For this review, take the finished solid that the model builds, in its own axes (mm). Face numbers are marked on the shaded views. A direction names the side the tool comes from. Round coordinates to 2 decimals unless told otherwise and drop trailing zeros. Order: outer loops, then holes, each group sorted by start corner. A loop starts at its lowest first (then second) coordinate and runs counter-clockwise, first axis right, second up. Notation, with made-up numbers: (29, 42.5) -> (80, 42.5) arc R16 cw to (80, 64.5) -> close; hole circle Ø11 at (40, 48.25). An arc over 180 degrees is marked (long way). Answer in a Markdown table with one row per item.
```python
from build123d import *

# Parameters (mm, degrees)
SKIZZE1_W                       = 140
SKIZZE1_H                       = 210
AUFSATZ_LINEAR_AUSTRAGEN1_DEPTH = 2
SKIZZE2_W                       = 20
SKIZZE2_H                       = 210
AUFSATZ_LINEAR_AUSTRAGEN2_DEPTH = 15
SKIZZE3_W                       = 94.4
SKIZZE3_H                       = 56
SCHNITT_LINEAR_AUSTRAGEN1_DEPTH = 10
VERRUNDUNG1_R                   = 1


with BuildPart() as part:
    # Skizze1 → Aufsatz-Linear austragen1 (new body)
    with BuildSketch(Plane(origin=(0, 0, 0), x_dir=(1, 0, 0), z_dir=(0, 1, 0))):
        Rectangle(SKIZZE1_W, SKIZZE1_H)
    extrude(amount=AUFSATZ_LINEAR_AUSTRAGEN1_DEPTH)

    # Skizze2 → Aufsatz-Linear austragen2 (add)
    with BuildSketch(Plane(origin=(0, 2, 0), x_dir=(1, 0, 0), z_dir=(0, 1, 0))):
        with Locations((-46.2, 0)):
            Rectangle(SKIZZE2_W, SKIZZE2_H)
        with Locations((46.2, 0)):
            Rectangle(SKIZZE2_W, SKIZZE2_H)
    extrude(amount=AUFSATZ_LINEAR_AUSTRAGEN2_DEPTH)

    # Skizze3 → Schnitt-Linear austragen1 (cut)
    with BuildSketch(Plane(origin=(0, 17, 0), x_dir=(1, 0, 0), z_dir=(0, 1, 0))):
        Rectangle(SKIZZE3_W, SKIZZE3_H)
        with Locations((0, -68)):
            Rectangle(SKIZZE3_W, SKIZZE3_H)
        with Locations((0, 68)):
            Rectangle(SKIZZE3_W, SKIZZE3_H)
    extrude(amount=-SCHNITT_LINEAR_AUSTRAGEN1_DEPTH, mode=Mode.SUBTRACT)

    # Verrundung1
    verrundung1_edges = [part.edges().sort_by_distance(p)[0] for p in [
        (41.7, 17, 28),
        (41.7, 17, -40),
        (41.7, 17, 96),
        (36.2, 7, 0),
        (36.2, 7, -68),
        (36.2, 7, 68),
        (-36.2, 7, 68),
        (-41.7, 17, 40),
        (-47.2, 17, 68),
        (-41.7, 17, 96),
        (47.2, 17, 68),
        (41.7, 17, 40),
        (-36.2, 12, 96),
        (36.2, 12, 96),
        (-36.2, 12, 40),
        (36.2, 12, 40),
        (-36.2, 7, -68),
        (-41.7, 17, -96),
        (-47.2, 17, -68),
        (-41.7, 17, -40),
        (47.2, 17, -68),
        (41.7, 17, -96),
        (-36.2, 12, -40),
        (36.2, 12, -40),
        (-36.2, 12, -96),
        (36.2, 12, -96),
        (-36.2, 7, 0),
        (-41.7, 17, -28),
        (-47.2, 17, 0),
        (-41.7, 17, 28),
        (47.2, 17, 0),
        (41.7, 17, -28),
        (-36.2, 12, 28),
        (36.2, 12, 28),
        (-36.2, 12, -28),
        (36.2, 12, -28),
    ]]
    fillet(verrundung1_edges, radius=VERRUNDUNG1_R)


solid = part.part
```
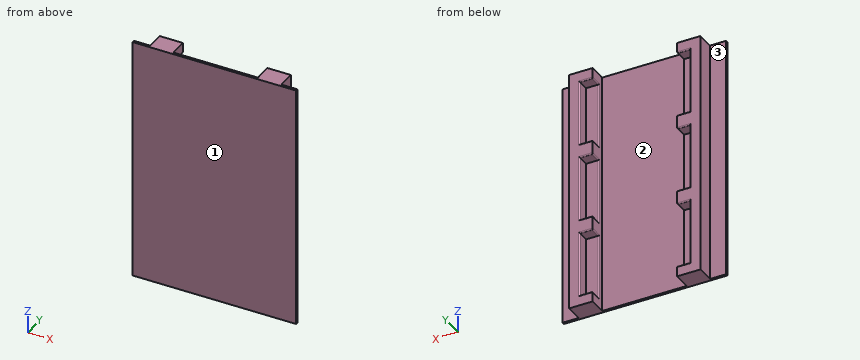
Q1. Clearance check with flat-ended pins moving along their axes: pin 1 Ø1 at (y, z) = (10, 57) entering from -X; pin 2 Ø7 at (y, z) = (9.5, -58.5) entering from +X; pin 3 Ø2 at (x, z) = (40.5, 73.5) entering from -Y; pin 4 Ø7 at (x, z) = (-61.5, -28.5) entering from +Y. State where each tip first meets the part, or that it passes through.
Answer key:
| item | result |
|---|---|
| pin 1 | stops at x = -56.2 |
| pin 2 | stops at x = 56.2 |
| pin 3 | stops at y = 0 |
| pin 4 | stops at y = 2 |
Q2. Tool access review of the marked faces 1, 2 and 3: name each direction out of +Z, -Z, +X, -X, +Y, -Y from which nothing blocks a thin tool from reaching the whole face with its end or side.
Answer key:
| item | result |
|---|---|
| face 1 | +Z, -Z, +X, -X, -Y |
| face 2 | +Z, -Z, +Y |
| face 3 | +Z, -Z, -X, +Y |
Q3. Take a section at B-B, the plane x = 15.5. Write out the cut boundary in (y, z).
Answer key:
| item | result |
|---|---|
| outline | (0, -105) -> (2, -105) -> (2, 105) -> (0, 105) -> close |
Q4. Take a section at A-A, the plane z = 51. Write out the cut boundary in (x, y), then the cut area to 3 significant figures.
Answer key:
| item | result |
|---|---|
| outline | (-70, 0) -> (70, 0) -> (70, 2) -> (56.2, 2) -> (56.2, 17) -> (48.2, 17) arc R1 ccw to (47.2, 16) -> (47.2, 7) -> (37.2, 7) arc R1 ccw to (36.2, 6) -> (36.2, 2) -> (-36.2, 2) -> (-36.2, 6) arc R1 ccw to (-37.2, 7) -> (-47.2, 7) -> (-47.2, 16) arc R1 ccw to (-48.2, 17) -> (-56.2, 17) -> (-56.2, 2) -> (-70, 2) -> close |
| area | 659 mm^2 |
Q5. To check wall thickness, follow probe 1 along Z at (x, y) = (-45.5, 10); probe 2 along X at (y, z) = (4, 39); probe 3 along X at (y, z) = (8, -9). State the ranges of each line that lie inside material, in increasing order.
Answer key:
| item | result |
|---|---|
| probe 1 | z = -105 to -96, -40 to -28, 28 to 40, 96 to 105 |
| probe 2 | x = -56.2 to -36.2, 36.2 to 56.2 |
| probe 3 | x = -56.2 to -47.2, 47.2 to 56.2 |
